Can you work these out from the model? Positions are in its coordinate system, mm. Give positions to 0.01 mm unless a question says otherwise; leave off trailing zeros. Order: outer loops, then holes, each group sorted by start corner. A loop starts at its lowest first (then second) coordinate and runs counter-clockwise, first axis right, second up. Notation, with made-up numbers: M 37.25,-37 L 58.25,-37 A25 cw 58.25,-17 Z; hole C 50.5,4.25 d5. An arc over 180 degrees is marked long. Use one line per item in the form item = value. Start each with the question number.
1. I need wall thicknesses on L1, parallel to Z at x = -0.75, y = 1.1; L2, parallel to Z at x = -1.05, y = -0.25; L3, parallel to Y at x = -0.05, z = 8.25. Which ranges of each line are inside material? Lowest first, please.
2. We'd pull the mould along Y, two halves only. Please class faces 1 (the face through (-0.91, -0.7, 7.07)), 2 (the face through (0, 0, 13)), 3 (the face through (0, 0, 1)): +Y half, -Y half, draft (parallel to the pull), parting line (faces both ways), or undercut.
3. I want a section at A-A, the plane y = 0. List the corners of the cut face in (x, z) for me.
4. I want a section at C-C, the plane z = 10.5. List the corners of the cut face in (x, y) for me, and give its area (3 significant figures).
5. Will these pins go through, and if not, where does the flat tip stop? P1, Ø0.6, axis at x = -0.5, z = 0.5, coming from the -Y side; P2, Ø0.6, axis at y = 1, z = 0.5, coming from the +X side.
```python
from build123d import *

# Parameters (mm, degrees)
SKETCH1_R           = 1.95
BOSS_EXTRUDE1_DEPTH = 1.3
CUT_EXTRUDE1_DEPTH  = 1
SKETCH3_R           = 1.15
BOSS_EXTRUDE2_DEPTH = 11.7
FILLET1_R           = 0.5


with BuildPart() as part:
    # Sketch1 → Boss-Extrude1 (new body)
    with BuildSketch(Plane.XY):
        Circle(SKETCH1_R)
    extrude(amount=BOSS_EXTRUDE1_DEPTH)

    # Sketch2 → Cut-Extrude1 (cut)
    with BuildSketch(Plane(origin=(0, 0, 0), x_dir=(-1, 0, 0), z_dir=(0, 0, -1))):
        with BuildLine():
            Line((-0.15, 1.25), (0.15, 1.25))
            ThreePointArc((0.15, 1.25), (0.291421356, 1.191421356), (0.35, 1.05))
            Line((0.35, 1.05), (0.35, 0.55))
            ThreePointArc((0.35, 0.55), (0.408578644, 0.408578644), (0.55, 0.35))
            Line((0.55, 0.35), (1.05, 0.35))
            ThreePointArc((1.05, 0.35), (1.191421356, 0.291421356), (1.25, 0.15))
            Line((1.25, 0.15), (1.25, -0.15))
            ThreePointArc((1.25, -0.15), (1.191421356, -0.291421356), (1.05, -0.35))
            Line((1.05, -0.35), (0.55, -0.35))
            ThreePointArc((0.55, -0.35), (0.408578644, -0.408578644), (0.35, -0.55))
            Line((0.35, -0.55), (0.35, -1.05))
            ThreePointArc((0.35, -1.05), (0.291421356, -1.191421356), (0.15, -1.25))
            Line((0.15, -1.25), (-0.15, -1.25))
            ThreePointArc((-0.15, -1.25), (-0.291421356, -1.191421356), (-0.35, -1.05))
            Line((-0.35, -1.05), (-0.35, -0.55))
            ThreePointArc((-0.35, -0.55), (-0.408578644, -0.408578644), (-0.55, -0.35))
            Line((-0.55, -0.35), (-1.05, -0.35))
            ThreePointArc((-1.05, -0.35), (-1.191421356, -0.291421356), (-1.25, -0.15))
            Line((-1.25, -0.15), (-1.25, 0.15))
            ThreePointArc((-1.25, 0.15), (-1.191421356, 0.291421356), (-1.05, 0.35))
            Line((-1.05, 0.35), (-0.55, 0.35))
            ThreePointArc((-0.55, 0.35), (-0.408578644, 0.408578644), (-0.35, 0.55))
            Line((-0.35, 0.55), (-0.35, 1.05))
            ThreePointArc((-0.35, 1.05), (-0.291421356, 1.191421356), (-0.15, 1.25))
        make_face()
    extrude(amount=-CUT_EXTRUDE1_DEPTH, mode=Mode.SUBTRACT)

    # Sketch3 → Boss-Extrude2 (add)
    with BuildSketch(Plane.XY.offset(1.3)):
        Circle(SKETCH3_R)
    extrude(amount=BOSS_EXTRUDE2_DEPTH)

    # Fillet1
    fillet1_edges = [part.edges().sort_by_distance(p)[0] for p in [
        (-1.95, 0, 0),
        (-1.95, 0, 1.3),
    ]]
    fillet(fillet1_edges, radius=FILLET1_R)


solid = part.part
```
Check result:
q1.L1 = 0 to 1.3
q1.L2 = 1 to 13
q1.L3 = -1.15 to 1.15
q2.face_1 = parting line
q2.face_2 = draft
q2.face_3 = undercut
q3.outline = M -1.95,0.5 A0.5 ccw -1.45,0 L -1.25,0 L -1.25,1 L 1.25,1 L 1.25,0 L 1.45,0 A0.5 ccw 1.95,0.5 L 1.95,0.8 A0.5 ccw 1.45,1.3 L 1.15,1.3 L 1.15,13 L -1.15,13 L -1.15,1.3 L -1.45,1.3 A0.5 ccw -1.95,0.8 Z
q4.outline = C 0,0 d2.3
q4.area = 4.15 mm2
q5.P1 = -1.94
q5.P2 = 1.82
